Source: CAD feature listing. Evaluate the final solid. Frame: model axes, mm. Face numbers are marked on the shaded views. Round coordinates to 2 decimals unless told otherwise and drop trailing zeros. Order: outer loops, then holes, each group sorted by start corner. A loop starts at its lowest first (then second) coordinate and runs counter-clockwise, first axis right, second up.
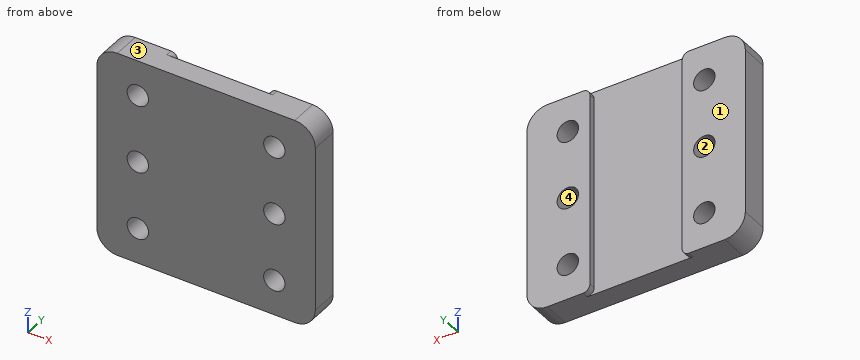
```python
from build123d import *

# Parameters (mm, degrees)
SKETCH1_W           = 50.8
SKETCH1_H           = 48.26
SKETCH1_R           = 2.4892
BOSS_EXTRUDE1_DEPTH = 3.175
FILLET1_R           = 4.7625
SKETCH3_W           = 21.450000026
SKETCH3_H           = 48.26
CUT_EXTRUDE2_DEPTH  = 1.499999794
FILLET2_R           = 1.600000102


with BuildPart() as part:
    # Sketch1 → Boss-Extrude1 (new, symmetric)
    with BuildSketch(Plane(origin=(0, 0, 0), x_dir=(1, 0, 0), z_dir=(0, 1, 0))):
        with Locations((25.4, 24.13)):
            Rectangle(SKETCH1_W, SKETCH1_H)
        with Locations(Location((9.525, 8.255, 0), (0, 0, 270))):
            Circle(SKETCH1_R, mode=Mode.SUBTRACT)
        with Locations(Location((9.525, 24.13, 0), (0, 0, 270))):
            Circle(SKETCH1_R, mode=Mode.SUBTRACT)
        with Locations(Location((9.525, 40.005, 0), (0, 0, 270))):
            Circle(SKETCH1_R, mode=Mode.SUBTRACT)
        with Locations(Location((41.275, 24.13, 0), (0, 0, 270))):
            Circle(SKETCH1_R, mode=Mode.SUBTRACT)
        with Locations(Location((41.275, 40.005, 0), (0, 0, 270))):
            Circle(SKETCH1_R, mode=Mode.SUBTRACT)
        with Locations(Location((41.275, 8.255, 0), (0, 0, 270))):
            Circle(SKETCH1_R, mode=Mode.SUBTRACT)
    extrude(amount=BOSS_EXTRUDE1_DEPTH, both=True)

    # Fillet1
    fillet1_edges = [part.edges().sort_by_distance(p)[0] for p in [
        (0, 0, 0),
        (0, 0, -48.26),
        (50.8, 0, -48.26),
        (50.8, 0, 0),
    ]]
    fillet(fillet1_edges, radius=FILLET1_R)

    # Sketch3 → Cut-Extrude2 (cut)
    with BuildSketch(Plane(origin=(0, 3.175, 0), x_dir=(1, 0, 0), z_dir=(0, 1, 0))):
        with Locations((25.4, 24.13)):
            Rectangle(SKETCH3_W, SKETCH3_H)
    extrude(amount=-CUT_EXTRUDE2_DEPTH, mode=Mode.SUBTRACT)

    # Fillet2
    fillet2_edges = [part.edges().sort_by_distance(p)[0] for p in [
        (14.674999987, 2.425000103, 0),
        (14.674999987, 2.425000103, -48.26),
        (36.125000013, 2.425000103, -48.26),
        (36.125000013, 2.425000103, 0),
    ]]
    fillet(fillet2_edges, radius=FILLET2_R)


solid = part.part
```
1. Section B-B on x = 10.5. Return loops of the section in (y, z) (3 decimals).
2. Section C-C on z = -12. Return loops of the section in (x, y) (3 decimals), plus the area to 3 significant figures.
3. Section A-A on z = -24.13. Return loops of the section in (x, y) (3 decimals), plus the area to 3 significant figures.
4. First-contact query: pin 1 (4.5 mm diameter, centred on x = 9.525, z = -40.005, fed in from +Y). Flat tip, straight axial feed; report the tip coordinate or a pass-through.
5. Section D-D on y = -2. Return loops of the section in (x, z) (1 decimal), plus the area to 3 significant figures.
6. Pull-direction query (Z, two-part tool) for the marked faces 1, 2, 3 and 4; classes: released by +Z, released by -Z, zero draft, split by the parting line, or undercut.
7. Line query: line 1 along X through (y, z) = (-0.5, -40); line 2 along Z through (x, y) = (41.5, 1.5); line 3 along X through (y, z) = (2.25, -41) (3 decimals). Output: solid intervals per line, ascending.
Result:
1. outline: (-3.175, -48.26) - (3.175, -48.26) - (3.175, -42.295) - (-3.175, -42.295) - close; (-3.175, -37.715) - (3.175, -37.715) - (3.175, -26.42) - (-3.175, -26.42) - close; (-3.175, -21.84) - (3.175, -21.84) - (3.175, -10.545) - (-3.175, -10.545) - close; (-3.175, -5.965) - (3.175, -5.965) - (3.175, 0) - (-3.175, 0) - close
2. outline: (0, -3.175) - (50.8, -3.175) - (50.8, 3.175) - (36.125, 3.175) - (36.125, 1.675) - (14.675, 1.675) - (14.675, 3.175) - (0, 3.175) - close
2. area: 290 mm2
3. outline: (0, -3.175) - (7.036, -3.175) - (7.036, 3.175) - (0, 3.175) - close; (12.014, -3.175) - (38.786, -3.175) - (38.786, 3.175) - (36.125, 3.175) - (36.125, 1.675) - (14.675, 1.675) - (14.675, 3.175) - (12.014, 3.175) - close; (43.764, -3.175) - (50.8, -3.175) - (50.8, 3.175) - (43.764, 3.175) - close
3. area: 227 mm2
4. pin 1: passes through
5. outline: (0, -43.5) arc R4.8 ccw to (4.8, -48.3) - (46, -48.3) arc R4.8 ccw to (50.8, -43.5) - (50.8, -4.8) arc R4.8 ccw to (46, 0) - (4.8, 0) arc R4.8 ccw to (0, -4.8) - close; hole circle Ø5 at (9.5, -40); hole circle Ø5 at (9.5, -24.1); hole circle Ø5 at (9.5, -8.3); hole circle Ø5 at (41.3, -40); hole circle Ø5 at (41.3, -24.1); hole circle Ø5 at (41.3, -8.3)
5. area: 2,320 mm2
6. face 1: zero draft
6. face 2: undercut
6. face 3: released by +Z
6. face 4: undercut
7. line 1: x = 0 to 7.04, 12.01 to 38.79, 43.76 to 50.8
7. line 2: z = -48.26 to -42.48, -37.53 to -26.61, -21.65 to -10.73, -5.78 to 0
7. line 3: x = 0 to 7.243, 11.807 to 14.675, 36.125 to 38.993, 43.557 to 50.8
